Input: dimensioned drawing with shaded views. Units: mm. Origin: part minimum x, y, z. Coordinates: 2 decimals unless noted, no trailing zeros. Order: outer loops, then holes, each group sorted by start corner. A loop starts at its lowest first (then second) coordinate and runs counter-clockwise, first axis right, second up.
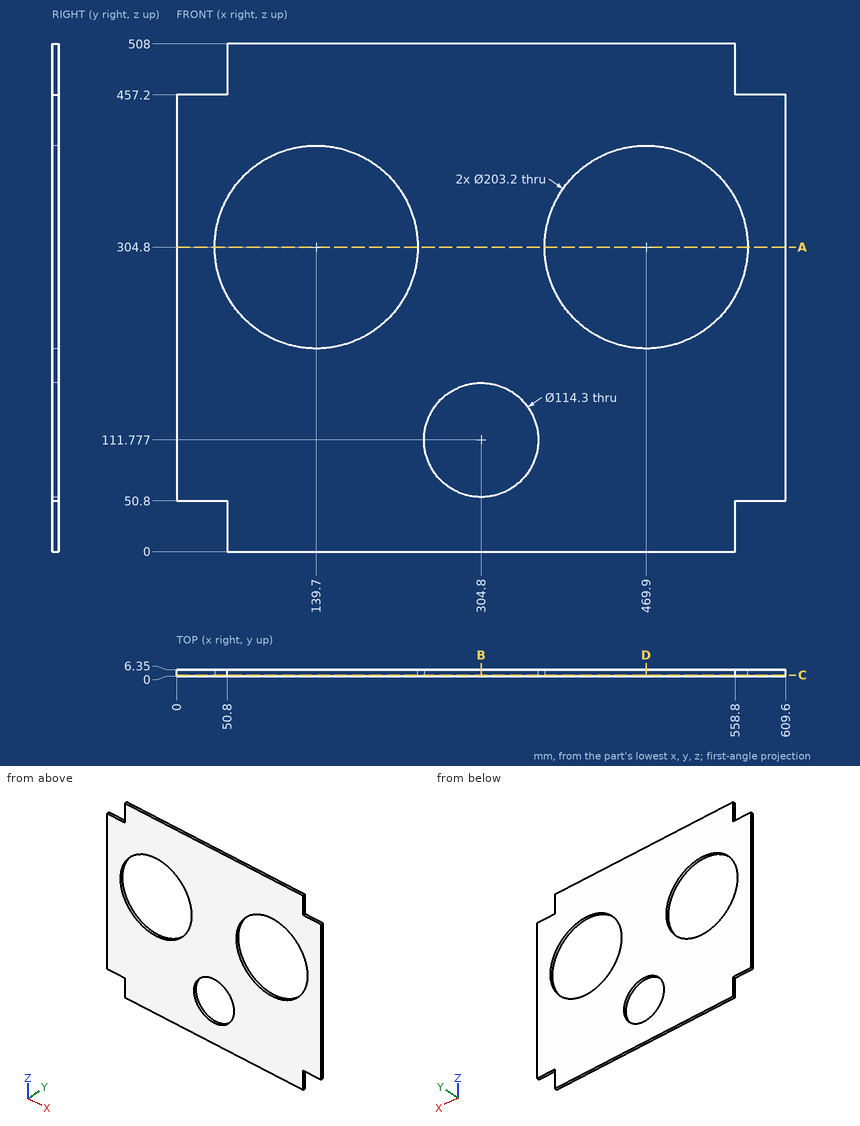
1. Pin query (flat end, axial travel): P1, Ø1.9, axis at x = 16.5, y = 3.5, coming from the -Z side; P2, Ø1.9, axis at y = 4.5, z = 480, coming from the -X side. Return the tip coordinate at first contact, or that it passes through.
Findings:
P1: stops at z = 50.8
P2: stops at x = 50.8
2. Section query C-C on y = 1. Return loops of the section in (x, z).
Findings:
outline: (0, 50.8) - (50.8, 50.8) - (50.8, 0) - (558.8, 0) - (558.8, 50.8) - (609.6, 50.8) - (609.6, 457.2) - (558.8, 457.2) - (558.8, 508) - (50.8, 508) - (50.8, 457.2) - (0, 457.2) - close; hole circle Ø203.2 at (139.7, 304.8); hole circle Ø114.3 at (304.8, 111.78); hole circle Ø203.2 at (469.9, 304.8)
3. Section query D-D on x = 469.9. Return loops of the section in (y, z).
Findings:
outline: (0, 0) - (6.35, 0) - (6.35, 203.2) - (0, 203.2) - close; (0, 406.4) - (6.35, 406.4) - (6.35, 508) - (0, 508) - close
4. Section query B-B on x = 304.8. Return loops of the section in (y, z), plus the area to 3 significant figures.
Findings:
outline: (0, 0) - (6.35, 0) - (6.35, 54.63) - (0, 54.63) - close; (0, 168.93) - (6.35, 168.93) - (6.35, 508) - (0, 508) - close
area: 2,500 mm2
5. Section query A-A on z = 304.8. Return loops of the section in (x, y), plus the area to 3 significant figures.
Findings:
outline: (0, 0) - (38.1, 0) - (38.1, 6.35) - (0, 6.35) - close; (241.3, 0) - (368.3, 0) - (368.3, 6.35) - (241.3, 6.35) - close; (571.5, 0) - (609.6, 0) - (609.6, 6.35) - (571.5, 6.35) - close
area: 1,290 mm2
6. Ray query, line 1 (X direction, y = 5, z = 304.8); line 2 (Z direction, x = 139.7, y = 2.5); line 3 (X direction, y = 3, z = 115.5). Return the intervals inside material, ascending.
Findings:
line 1: x = 0 to 38.1, 241.3 to 368.3, 571.5 to 609.6
line 2: z = 0 to 203.2, 406.4 to 508
line 3: x = 0 to 247.77, 361.83 to 609.6
